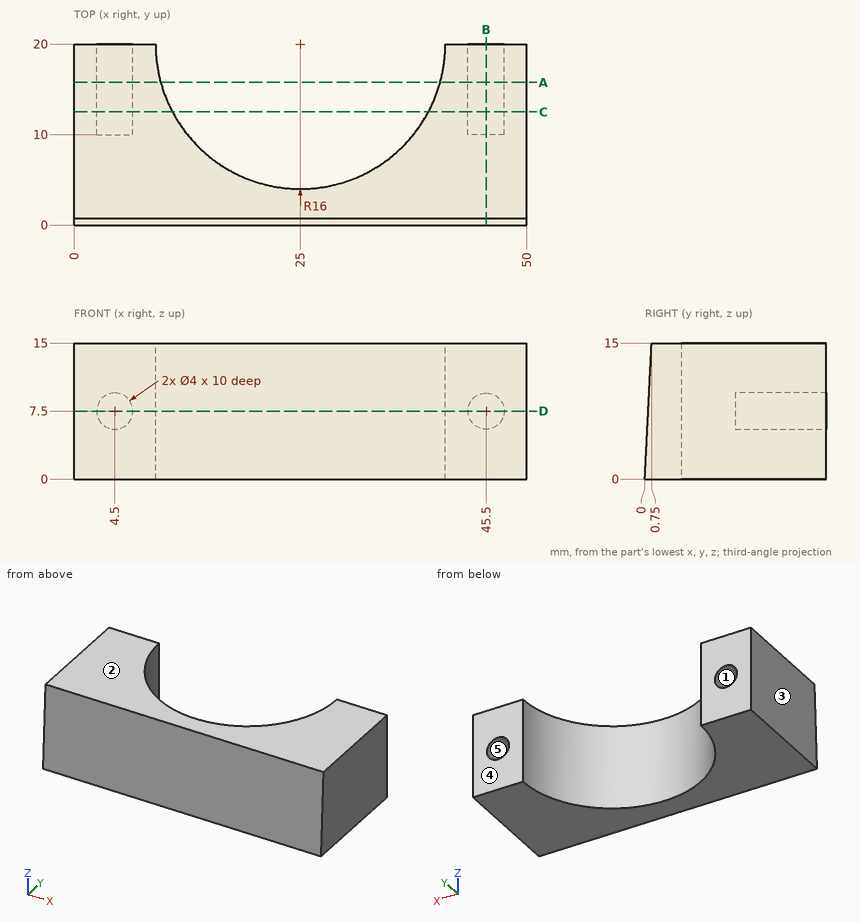
The figure shows three views and two pictorial views of one solid part (mm, origin at its lowest corner). Answer the questions. A direction names the side the tool comes from. Coordinates: 2 decimals unless noted, no trailing zeros. Loops run counter-clockwise (first coordinate to the right, second up) from the corner with the lowest first, then second, coordinate; pieces in that order, holes last.
1) Determine the mould class of the marked faces 3, 4 and 5 for opening direction X: pulls with the +X half, pulls with the -X half, needs draft (parallel to the pull), parting line crosses it, or undercut.
2) Find the intervals of material crossed by L1, parallel to X at y = 17.5, z = 7.5; L2, parallel to X at y = 15.25, z = 7.5; L3, parallel to X at y = 7.5, z = 12.5, in increasing order.
3) Find section A-A on y = 15.75. Write down the section's boundary in (x, z), then the cut area to 3 significant figures.
4) Find section C-C on y = 12.5. Write down the section's boundary in (x, z), then the cut area to 3 significant figures.
5) Find section D-D on z = 7.5. Write down the section's boundary in (x, y) (3 decimals).
6) A tool of negligible diameter and unlimited length cuts with its end or side. For the marked faces 1 and 2, from which of +Z, -Z, +X, -X, +Y, -Y can it reach the whole face along a straight path? Write none if from no direction.
7) Find section B-B on x = 45.5. Write down the section's boundary in (y, z), then the cut area to 3 significant figures.
8) Flat-ended cylindrical pins translate along their axes: pin 1 Ø2 at (y, z) = (12.5, 13) entering from -X; pin 2 Ø2 at (x, z) = (45, 7.5) entering from +Y; pin 3 Ø5 at (x, z) = (44, 6) entering from -Y (3 decimals); pin 4 Ø3.5 at (x, z) = (45.5, 7.5) entering from -Y. Find the tip coordinate at first contact, or state that the pin passes through.
Values:
1. face 3: pulls with the -X half
1. face 4: needs draft
1. face 5: undercut
2. L1: x = 0 to 2.5, 6.5 to 9.2, 40.8 to 43.5, 47.5 to 50
2. L2: x = 0 to 2.5, 6.5 to 9.72, 40.28 to 43.5, 47.5 to 50
2. L3: x = 0 to 15.01, 34.99 to 50
3. outline: (0, 0) - (9.57, 0) - (9.57, 15) - (0, 15) - close; (40.43, 0) - (50, 0) - (50, 15) - (40.43, 15) - close; hole circle Ø4 at (4.5, 7.5); hole circle Ø4 at (45.5, 7.5)
3. area: 262 mm2
4. outline: (0, 0) - (10.87, 0) - (10.87, 15) - (0, 15) - close; (39.13, 0) - (50, 0) - (50, 15) - (39.13, 15) - close; hole circle Ø4 at (4.5, 7.5); hole circle Ø4 at (45.5, 7.5)
4. area: 301 mm2
5. outline: (0, 0.375) - (50, 0.375) - (50, 20) - (47.5, 20) - (47.5, 10) - (43.5, 10) - (43.5, 20) - (41, 20) arc R16 cw to (9, 20) - (6.5, 20) - (6.5, 10) - (2.5, 10) - (2.5, 20) - (0, 20) - close
6. face 1: +Y
6. face 2: +Z, +X, -X, +Y, -Y
7. outline: (0, 0) - (20, 0) - (20, 5.5) - (10, 5.5) - (10, 9.5) - (20, 9.5) - (20, 15) - (0.75, 15) - close
7. area: 254 mm2
8. pin 1: stops at x = 0
8. pin 2: stops at y = 10
8. pin 3: stops at y = 0.175
8. pin 4: stops at y = 0.29
